from build123d import *

# Parameters (mm, degrees)
SKETCH1_W                    = 33
SKETCH1_H                    = 55
BOSS_EXTRUDE1_DEPTH          = 4
SKETCH2_W                    = 33
SKETCH2_H                    = 5
BOSS_EXTRUDE2_DEPTH          = 20
CUT_EXTRUDE1_REACH           = 69.186
SKETCH3_R                    = 1.25
SKETCH3_R_2                  = 5.6
M3_START                     = -55
M3_CLEARANCE_HOLE1_OUTLINE_R = 1.7
M3_CLEARANCE_HOLE1_DEPTH     = 5


# Read off the part's stored shape, not the designer's step: M3 Clearance Hole1
with BuildPart() as part:
    # Sketch1 → Boss-Extrude1 (new body)
    with BuildSketch(Plane.XY):
        with Locations((16.5, -27.5)):
            Rectangle(SKETCH1_W, SKETCH1_H)
    extrude(amount=BOSS_EXTRUDE1_DEPTH)

    # Sketch2 → Boss-Extrude2 (add)
    with BuildSketch(Plane.XY.offset(4)):
        with Locations((16.5, -52.5)):
            Rectangle(SKETCH2_W, SKETCH2_H)
    extrude(amount=BOSS_EXTRUDE2_DEPTH)

    # Sketch3 → Cut-Extrude1 (cut, up to next)
    with BuildSketch(Plane.XY.offset(4), mode=Mode.PRIVATE) as cut_extrude1_sk1:
        with Locations((30.1, -9.57)):
            Circle(SKETCH3_R)
    cut_extrude1_tool1 = extrude(cut_extrude1_sk1.sketch, amount=-CUT_EXTRUDE1_REACH, mode=Mode.PRIVATE) & part.part
    # Sketch3 → Cut-Extrude1 (cut, up to next)
    with BuildSketch(Plane.XY.offset(4), mode=Mode.PRIVATE) as cut_extrude1_sk2:
        with Locations((30.1, -17.57)):
            Circle(SKETCH3_R)
    cut_extrude1_tool2 = extrude(cut_extrude1_sk2.sketch, amount=-CUT_EXTRUDE1_REACH, mode=Mode.PRIVATE) & part.part
    # Sketch3 → Cut-Extrude1 (cut, up to next)
    with BuildSketch(Plane.XY.offset(4), mode=Mode.PRIVATE) as cut_extrude1_sk3:
        with Locations((30.1, -25.57)):
            Circle(SKETCH3_R)
    cut_extrude1_tool3 = extrude(cut_extrude1_sk3.sketch, amount=-CUT_EXTRUDE1_REACH, mode=Mode.PRIVATE) & part.part
    # Sketch3 → Cut-Extrude1 (cut, up to next)
    with BuildSketch(Plane.XY.offset(4), mode=Mode.PRIVATE) as cut_extrude1_sk4:
        with Locations((30.1, -33.57)):
            Circle(SKETCH3_R)
    cut_extrude1_tool4 = extrude(cut_extrude1_sk4.sketch, amount=-CUT_EXTRUDE1_REACH, mode=Mode.PRIVATE) & part.part
    # Sketch3 → Cut-Extrude1 (cut, up to next)
    with BuildSketch(Plane.XY.offset(4), mode=Mode.PRIVATE) as cut_extrude1_sk5:
        with Locations((3.1, -33.57)):
            Circle(SKETCH3_R)
    cut_extrude1_tool5 = extrude(cut_extrude1_sk5.sketch, amount=-CUT_EXTRUDE1_REACH, mode=Mode.PRIVATE) & part.part
    # Sketch3 → Cut-Extrude1 (cut, up to next)
    with BuildSketch(Plane.XY.offset(4), mode=Mode.PRIVATE) as cut_extrude1_sk6:
        with Locations((3.1, -25.57)):
            Circle(SKETCH3_R)
    cut_extrude1_tool6 = extrude(cut_extrude1_sk6.sketch, amount=-CUT_EXTRUDE1_REACH, mode=Mode.PRIVATE) & part.part
    # Sketch3 → Cut-Extrude1 (cut, up to next)
    with BuildSketch(Plane.XY.offset(4), mode=Mode.PRIVATE) as cut_extrude1_sk7:
        with Locations((3.1, -17.57)):
            Circle(SKETCH3_R)
    cut_extrude1_tool7 = extrude(cut_extrude1_sk7.sketch, amount=-CUT_EXTRUDE1_REACH, mode=Mode.PRIVATE) & part.part
    # Sketch3 → Cut-Extrude1 (cut, up to next)
    with BuildSketch(Plane.XY.offset(4), mode=Mode.PRIVATE) as cut_extrude1_sk8:
        with Locations((3.1, -9.57)):
            Circle(SKETCH3_R)
    cut_extrude1_tool8 = extrude(cut_extrude1_sk8.sketch, amount=-CUT_EXTRUDE1_REACH, mode=Mode.PRIVATE) & part.part
    # Sketch3 → Cut-Extrude1 (cut, up to next)
    with BuildSketch(Plane.XY.offset(4), mode=Mode.PRIVATE) as cut_extrude1_sk9:
        with Locations((8.6, -4.32)):
            Circle(SKETCH3_R)
    cut_extrude1_tool9 = extrude(cut_extrude1_sk9.sketch, amount=-CUT_EXTRUDE1_REACH, mode=Mode.PRIVATE) & part.part
    # Sketch3 → Cut-Extrude1 (cut, up to next)
    with BuildSketch(Plane.XY.offset(4), mode=Mode.PRIVATE) as cut_extrude1_sk10:
        with Locations((24.6, -4.32)):
            Circle(SKETCH3_R)
    cut_extrude1_tool10 = extrude(cut_extrude1_sk10.sketch, amount=-CUT_EXTRUDE1_REACH, mode=Mode.PRIVATE) & part.part
    # Sketch3 → Cut-Extrude1 (cut, up to next)
    with BuildSketch(Plane.XY.offset(4), mode=Mode.PRIVATE) as cut_extrude1_sk11:
        with Locations((16.6, -40.32)):
            Circle(SKETCH3_R_2)
    cut_extrude1_tool11 = extrude(cut_extrude1_sk11.sketch, amount=-CUT_EXTRUDE1_REACH, mode=Mode.PRIVATE) & part.part
    # Sketch3 → Cut-Extrude1 (cut, up to next)
    with BuildSketch(Plane.XY.offset(4), mode=Mode.PRIVATE) as cut_extrude1_sk12:
        with BuildLine():
            Line((6.9, -15.32), (12.3, -15.32))
            ThreePointArc((12.3, -15.32), (12.865685425, -15.085685425), (13.1, -14.52))
            Line((13.1, -14.52), (13.1, -8.12))
            ThreePointArc((13.1, -8.12), (12.865685425, -7.554314575), (12.3, -7.32))
            Line((12.3, -7.32), (6.9, -7.32))
            ThreePointArc((6.9, -7.32), (6.334314575, -7.554314575), (6.1, -8.12))
            Line((6.1, -8.12), (6.1, -14.52))
            ThreePointArc((6.1, -14.52), (6.334314575, -15.085685425), (6.9, -15.32))
        make_face()
    cut_extrude1_tool12 = extrude(cut_extrude1_sk12.sketch, amount=-CUT_EXTRUDE1_REACH, mode=Mode.PRIVATE) & part.part
    # Sketch3 → Cut-Extrude1 (cut, up to next)
    with BuildSketch(Plane.XY.offset(4), mode=Mode.PRIVATE) as cut_extrude1_sk13:
        with BuildLine():
            Line((27.1, -8.12), (27.1, -14.52))
            ThreePointArc((27.1, -14.52), (26.865685425, -15.085685425), (26.3, -15.32))
            Line((26.3, -15.32), (20.9, -15.32))
            ThreePointArc((20.9, -15.32), (20.334314575, -15.085685425), (20.1, -14.52))
            Line((20.1, -14.52), (20.1, -8.12))
            ThreePointArc((20.1, -8.12), (20.334314575, -7.554314575), (20.9, -7.32))
            Line((20.9, -7.32), (26.3, -7.32))
            ThreePointArc((26.3, -7.32), (26.865685425, -7.554314575), (27.1, -8.12))
        make_face()
    cut_extrude1_tool13 = extrude(cut_extrude1_sk13.sketch, amount=-CUT_EXTRUDE1_REACH, mode=Mode.PRIVATE) & part.part
    # Sketch3 → Cut-Extrude1 (cut, up to next)
    with BuildSketch(Plane.XY.offset(4), mode=Mode.PRIVATE) as cut_extrude1_sk14:
        Polygon((6.4, -21.42), (16.5, -21.42), (16.7, -21.42), (26.8, -21.42), (26.8, -28.72), (16.7, -28.72), (16.5, -28.72), (6.4, -28.72), align=None)
    cut_extrude1_tool14 = extrude(cut_extrude1_sk14.sketch, amount=-CUT_EXTRUDE1_REACH, mode=Mode.PRIVATE) & part.part
    add(cut_extrude1_tool1.solids().sort_by_distance((30.1, -9.57, 4))[0], mode=Mode.SUBTRACT)
    add(cut_extrude1_tool2.solids().sort_by_distance((30.1, -17.57, 4))[0], mode=Mode.SUBTRACT)
    add(cut_extrude1_tool3.solids().sort_by_distance((30.1, -25.57, 4))[0], mode=Mode.SUBTRACT)
    add(cut_extrude1_tool4.solids().sort_by_distance((30.1, -33.57, 4))[0], mode=Mode.SUBTRACT)
    add(cut_extrude1_tool5.solids().sort_by_distance((3.1, -33.57, 4))[0], mode=Mode.SUBTRACT)
    add(cut_extrude1_tool6.solids().sort_by_distance((3.1, -25.57, 4))[0], mode=Mode.SUBTRACT)
    add(cut_extrude1_tool7.solids().sort_by_distance((3.1, -17.57, 4))[0], mode=Mode.SUBTRACT)
    add(cut_extrude1_tool8.solids().sort_by_distance((3.1, -9.57, 4))[0], mode=Mode.SUBTRACT)
    add(cut_extrude1_tool9.solids().sort_by_distance((8.6, -4.32, 4))[0], mode=Mode.SUBTRACT)
    add(cut_extrude1_tool10.solids().sort_by_distance((24.6, -4.32, 4))[0], mode=Mode.SUBTRACT)
    add(cut_extrude1_tool11.solids().sort_by_distance((16.6, -40.32, 4))[0], mode=Mode.SUBTRACT)
    add(cut_extrude1_tool12.solids().sort_by_distance((9.6, -11.32, 4))[0], mode=Mode.SUBTRACT)
    add(cut_extrude1_tool13.solids().sort_by_distance((23.6, -11.32, 4))[0], mode=Mode.SUBTRACT)
    add(cut_extrude1_tool14.solids().sort_by_distance((16.6, -25.07, 4))[0], mode=Mode.SUBTRACT)

    # M3 Clearance Hole1 outline → M3 Clearance Hole1 (cut)
    with BuildSketch(Plane(origin=(0, 0, 0), x_dir=(1, 0, 0), z_dir=(0, 1, 0)).offset(M3_START)):
        with Locations((29, -8)):
            Circle(M3_CLEARANCE_HOLE1_OUTLINE_R)
        with Locations((4, -20)):
            Circle(M3_CLEARANCE_HOLE1_OUTLINE_R)
        with Locations((29, -20)):
            Circle(M3_CLEARANCE_HOLE1_OUTLINE_R)
        with Locations((4, -8)):
            Circle(M3_CLEARANCE_HOLE1_OUTLINE_R)
    extrude(amount=M3_CLEARANCE_HOLE1_DEPTH, mode=Mode.SUBTRACT)


solid = part.part
CAD build for the part. Positions are in the model's coordinates, mm. A direction names the side the tool comes from. Round coordinates to 2 decimals unless told otherwise and drop trailing zeros. Order: outer loops, then holes, each group sorted by start corner. A loop starts at its lowest first (then second) coordinate and runs counter-clockwise, first axis right, second up. Notation, with made-up numbers: (7, 6) - (30, 6) arc R24 ccw to (30, 29) - close; hole circle Ø9 at (-35.75, 3). An arc over 180 degrees is marked (long way). Return JSON: item names as keys, results as strings.
(1) Cut at B-B (y = -40.32). Give the cut face in (x, z).
Answer key:
{"outline": "(0, 0) - (11, 0) - (11, 4) - (0, 4) - close; (22.2, 0) - (33, 0) - (33, 4) - (22.2, 4) - close"}
(2) Cut at D-D (x = 3.1). State how many separate pieces and enclosed holes the cut face has, then the cut area to 3 significant figures.
Answer key:
{"separate pieces": "7", "enclosed holes": "0", "area": "251 mm^2"}
(3) Tool access for faces 1 (the face through (33, -36, 3)), 2 (the face through (26.8, -25, 2)): list every direction of +Z, -Z, +X, -X, +Y, -Y with a clear straight run to the whole face (end or side of a thin tool).
Answer key:
{"face 1": "+Z, -Z, +X, +Y, -Y", "face 2": "+Z, -Z"}
(4) Wall check: probe 1 along Y at (x, z) = (30.1, 1.7); probe 2 along X at (y, z) = (-52.5, 8); probe 3 along Z at (x, y) = (29, -52.4). Give the ranges that are in metal, low to high. Write a range as from..to.
Answer key:
{"probe 1": "y = -55..-34.82, -32.32..-26.82, -24.32..-18.82, -16.32..-10.82, -8.32..0", "probe 2": "x = 0..2.3, 5.7..27.3, 30.7..33", "probe 3": "z = 0..6.3, 9.7..18.3, 21.7..24"}
(5) Pull direction Y, two halves, no side cores. Call faces 3 (the face through (3.772, -16.516, 2.028)), 4 (the face through (24, -15.32, 2)), 5 (the face through (16, -33, 0)): +Y half, -Y half, draft (parallel to the pull), parting line (faces both ways), or undercut.
Answer key:
{"face 3": "undercut", "face 4": "undercut", "face 5": "draft"}
(6) Cut at A-A (z = 8). Give the cut face in (x, y), then the cut area to 3 significant figures.
Answer key:
{"outline": "(0, -55) - (2.3, -55) - (2.3, -50) - (0, -50) - close; (5.7, -55) - (27.3, -55) - (27.3, -50) - (5.7, -50) - close; (30.7, -55) - (33, -55) - (33, -50) - (30.7, -50) - close", "area": "131 mm^2"}
(7) Pin check, flat tips, straight feed: pin 1 Ø2 at (x, y) = (24.6, -4.32) entering from -Z; pin 2 Ø3 at (x, y) = (30.1, -33.57) entering from +Z; pin 3 Ø10 at (x, z) = (16.5, 19) entering from +Y. Stop position of each tip, or through.
Answer key:
{"pin 1": "passes through", "pin 2": "stops at z = 4", "pin 3": "stops at y = -50"}
(8) Cut at C-C (x = 16.6). Give the cut face in (y, z).
Answer key:
{"outline": "(-55, 0) - (-45.92, 0) - (-45.92, 4) - (-50, 4) - (-50, 24) - (-55, 24) - close; (-34.72, 0) - (-28.72, 0) - (-28.72, 4) - (-34.72, 4) - close; (-21.42, 0) - (0, 0) - (0, 4) - (-21.42, 4) - close"}
